from build123d import *

# Parameters (mm, degrees)
SKETCH1_R           = 2.5
BOSS_EXTRUDE1_DEPTH = 5


with BuildPart() as part:
    # Sketch1 → Boss-Extrude1 (new body)
    with BuildSketch(Plane.XY):
        with BuildLine():
            Line((-15, -5), (15, -5))
            Line((15, -5), (15, 40))
            Line((15, 40), (-20, 40))
            ThreePointArc((-20, 40), (-23.535533906, 38.535533906), (-25, 35))
            ThreePointArc((-25, 35), (-24.472135955, 32.763932023), (-23, 31))
            Line((-23, 31), (-15, 25))
            Line((-15, 25), (-15, -5))
        make_face()
        with Locations((-10, 0)):
            Circle(SKETCH1_R, mode=Mode.SUBTRACT)
        with Locations((10, 0)):
            Circle(SKETCH1_R, mode=Mode.SUBTRACT)
        with Locations((-20, 35)):
            Circle(SKETCH1_R, mode=Mode.SUBTRACT)
    extrude(amount=BOSS_EXTRUDE1_DEPTH)


solid = part.part
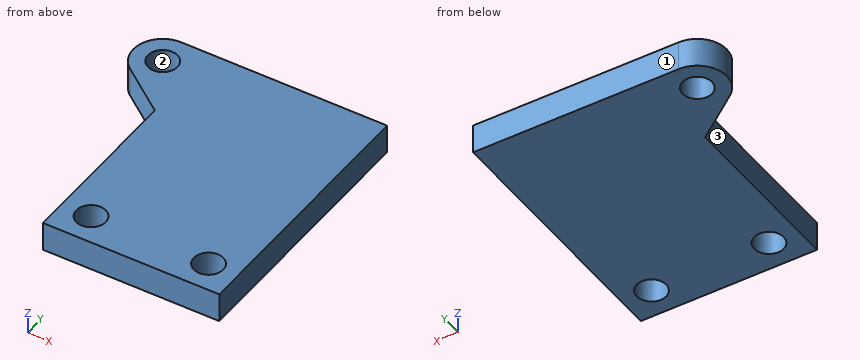
Here's how the part is built. I have some questions about the finished solid (model axes, mm). Face numbers are marked on the shaded views. Coordinates: 2 decimals unless noted, no trailing zeros. Loops run counter-clockwise (first coordinate to the right, second up) from the corner with the lowest first, then second, coordinate; pieces in that order, holes last.
1. Imagine slicing it at A-A, the plane y = 0. Please give me the cut outline in (x, z).
2. Imagine slicing it at C-C, the plane x = -10. Please give me the cut outline in (y, z), and give its area (3 significant figures).
3. I need wall thicknesses on L1, parallel to Y at x = 10, z = 2.2; L2, parallel to X at y = -0.5, z = 2.3; L3, parallel to X at y = 18, z = 3.55. Which ranges of each line are inside material? Lowest first, please.
4. If we mould it in two halves opening along Y, with no side actions, what happens to the marked faces 1, 2 and 3? For each: pulls with the +Y half, pulls with the -Y half, needs draft (parallel to the pull), parting line crosses it, or undercut.
5. Imagine slicing it at B-B, the plane z = 1.15. Please give me the cut outline in (x, y).
6. For P1, Ø1.5, axis at y = 31, z = 2.5, coming from the -X side, with a flat end and sliding along its axis, tell me the tip position at first contact or that it passes through.
7. Imagine slicing it at D-D, the plane y = 33.5. Please give me the cut outline in (x, z).
Taken from the geometry:
1. outline: (-15, 0) - (-12.5, 0) - (-12.5, 5) - (-15, 5) - close; (-7.5, 0) - (7.5, 0) - (7.5, 5) - (-7.5, 5) - close; (12.5, 0) - (15, 0) - (15, 5) - (12.5, 5) - close
2. outline: (-5, 0) - (-2.5, 0) - (-2.5, 5) - (-5, 5) - close; (2.5, 0) - (40, 0) - (40, 5) - (2.5, 5) - close
2. area: 200 mm2
3. L1: y = -5 to -2.5, 2.5 to 40
3. L2: x = -15 to -12.45, -7.55 to 7.55, 12.45 to 15
3. L3: x = -15 to 15
4. face 1: pulls with the +Y half
4. face 2: undercut
4. face 3: needs draft
5. outline: (-23, 31) - (-15, 25) - (-15, -5) - (15, -5) - (15, 40) - (-20, 40) arc R5 ccw to start; hole circle Ø5 at (-20, 35); hole circle Ø5 at (-10, 0); hole circle Ø5 at (10, 0)
6. P1: stops at x = -23.8
7. outline: (-24.77, 0) - (-22, 0) - (-22, 5) - (-24.77, 5) - close; (-18, 0) - (15, 0) - (15, 5) - (-18, 5) - close
